Source: CAD feature listing. Evaluate the final solid. Frame: model axes, mm. A direction names the side the tool comes from. Give positions to 0.01 mm unless a question says otherwise; leave off trailing zeros. Order: outer loops, then holes, each group sorted by start corner. A loop starts at its lowest first (then second) coordinate and runs counter-clockwise, first axis right, second up. Notation, with made-up numbers: (10.5, 6.25) - (59.5, 6.25) arc R5 cw to (59.5, 14.25) - close; hole circle Ø7 at (78, 15.5). An arc over 180 degrees is marked (long way). One line per item, written item: value. Start each with the question number.
from build123d import *

# Parameters (mm, degrees)
SKETCH1_R           = 48.25
SKETCH1_R_2         = 36
BOSS_EXTRUDE6_DEPTH = 10
SKETCH21_R          = 2
CUT_EXTRUDE1_DEPTH  = 18
CIRPATTERN1_COUNT   = 8
SKETCH22_R          = 3.5
CUT_EXTRUDE2_DEPTH  = 4
CIRPATTERN2_COUNT   = 8
SKETCH23_R          = 48.25
BOSS_EXTRUDE7_DEPTH = 6
CUT_EXTRUDE3_START  = -6
SKETCH25_R          = 3.5
CUT_EXTRUDE3_DEPTH  = 6
CIRPATTERN4_COUNT   = 8


with BuildPart() as part:
    # Sketch1 → Boss-Extrude6 (new body)
    with BuildSketch(Plane(origin=(0, 0, 0), x_dir=(1, 0, 0), z_dir=(0, 1, 0))):
        with Locations(Location((0, 0, 0), (0, 0, 270))):
            Circle(SKETCH1_R)
        with Locations(Location((0, 0, 0), (0, 0, 270))):
            Circle(SKETCH1_R_2, mode=Mode.SUBTRACT)
    extrude(amount=BOSS_EXTRUDE6_DEPTH)

    # Sketch21 → Cut-Extrude1 (cut)
    with BuildSketch(Plane(origin=(0, 10, 0), x_dir=(1, 0, 0), z_dir=(0, 1, 0))):
        with Locations(Location((-42.5, 0, 0), (0, 0, 270))):
            Circle(SKETCH21_R)
    cut_extrude1 = extrude(amount=-CUT_EXTRUDE1_DEPTH, mode=Mode.SUBTRACT)

    # CirPattern1: Cut-Extrude1 ×8 about axis
    cirpattern1_axis = Axis((0, 0, 0), (0, 1, 0))
    for i in range(1, CIRPATTERN1_COUNT):
        add(cut_extrude1.rotate(cirpattern1_axis, i * 360 / CIRPATTERN1_COUNT), mode=Mode.SUBTRACT)

    # Sketch22 → Cut-Extrude2 (cut)
    with BuildSketch(Plane(origin=(0, 10, 0), x_dir=(1, 0, 0), z_dir=(0, 1, 0))):
        with Locations(Location((-42.5, 0, 0), (0, 0, 270))):
            Circle(SKETCH22_R)
    cut_extrude2 = extrude(amount=-CUT_EXTRUDE2_DEPTH, mode=Mode.SUBTRACT)

    # CirPattern2: Cut-Extrude2 ×8 about axis
    cirpattern2_axis = Axis((0, 0, 0), (0, 1, 0))
    for i in range(1, CIRPATTERN2_COUNT):
        add(cut_extrude2.rotate(cirpattern2_axis, i * 360 / CIRPATTERN2_COUNT), mode=Mode.SUBTRACT)

    # Sketch23 → Boss-Extrude7 (add)
    with BuildSketch(Plane(origin=(0, 10, 0), x_dir=(1, 0, 0), z_dir=(0, 1, 0))):
        with Locations(Location((0, 0, 0), (0, 0, 270))):
            Circle(SKETCH23_R)
    extrude(amount=BOSS_EXTRUDE7_DEPTH)

    # Sketch25 → Cut-Extrude3 (cut)
    with BuildSketch(Plane.XZ.offset(-10).offset(CUT_EXTRUDE3_START)):
        with Locations(Location((-42.5, 0, 0), (0, 0, 90))):
            Circle(SKETCH25_R)
    cut_extrude3 = extrude(amount=CUT_EXTRUDE3_DEPTH, mode=Mode.SUBTRACT)

    # CirPattern4: Cut-Extrude3 ×8 about axis
    cirpattern4_axis = Axis((0, 10, 0), (0, -1, 0))
    for i in range(1, CIRPATTERN4_COUNT):
        add(cut_extrude3.rotate(cirpattern4_axis, i * 360 / CIRPATTERN4_COUNT), mode=Mode.SUBTRACT)


solid = part.part
1. Section A-A on x = 0. Return the cut outline in (y, z), then the cut area to 3 significant figures.
2. Section B-B on z = 0. Return the cut outline in (x, y), then the cut area to 3 significant figures.
3. Set-up query: faces 4 (the flat face through (28, 6, -32)), 5 (the cylindrical face through (-0.923, 3.042, -44.274)), 6 (the cylindrical face through (10.81, 4.93, 34.34)). Return all of +Z, -Z, +X, -X, +Y, -Y with unobstructed straight access to the full face (end or side cutting, diameter ignored); none if empty.
4. Draft query along Z for faces 1 (the cylindrical face through (-47.103, 7.888, -10.46)), 2 (the flat face through (-36, 0, 7)), 3 (the flat face through (44, 6, -2)). Return one class per face: pulls with the +Z half, pulls with the -Z half, needs draft (parallel to the pull), parting line crosses it, or undercut.
5. Section D-D on y = 12.5. Count the separate pieces of the cut face and the enclosed holes in it, then the cut area to 3 significant figures.
6. Ray query, L1, parallel to X at y = 7, z = 31.5; L2, parallel to Z at x = 2.5, y = 2.5; L3, parallel to Z at x = -27, y = 4.5. Return the intervals inside material, ascending.
7. Section C-C on z = 42.5. Return the cut outline in (x, y), then the cut area to 3 significant figures.
8. Contact query for flat-ended pins moving along their axis: pin 1 Ø5.5 at (x, z) = (0.5, -42) entering from +Y; pin 2 Ø1.5 at (x, y) = (-29, 14.5) entering from +Z; pin 3 Ø4 at (y, z) = (14, -23) entering from -X. Output: stop coordinate, or through.
Data:
1. outline: (0, -48.25) - (16, -48.25) - (16, -46) - (6, -46) - (6, -44.5) - (0, -44.5) - close; (0, -40.5) - (6, -40.5) - (6, -39) - (16, -39) - (16, 39) - (6, 39) - (6, 40.5) - (0, 40.5) - (0, 36) - (10, 36) - (10, -36) - (0, -36) - close; (0, 44.5) - (6, 44.5) - (6, 46) - (16, 46) - (16, 48.25) - (0, 48.25) - close
1. area: 636 mm2
2. outline: (-48.25, 0) - (-44.5, 0) - (-44.5, 6) - (-46, 6) - (-46, 16) - (-48.25, 16) - close; (-40.5, 0) - (-36, 0) - (-36, 10) - (36, 10) - (36, 0) - (40.5, 0) - (40.5, 6) - (39, 6) - (39, 16) - (-39, 16) - (-39, 6) - (-40.5, 6) - close; (44.5, 0) - (48.25, 0) - (48.25, 16) - (46, 16) - (46, 6) - (44.5, 6) - close
2. area: 636 mm2
3. face 4: +Y
3. face 5: +Y, -Y
3. face 6: -Y
4. face 1: parting line crosses it
4. face 2: needs draft
4. face 3: undercut
5. separate pieces: 1
5. enclosed holes: 8
5. area: 7,010 mm2
6. L1: x = -36.55 to -33.24, -26.87 to -17.43, 17.43 to 26.87, 33.24 to 36.55
6. L2: z = -48.19 to -35.91, 35.91 to 48.19
6. L3: z = -39.99 to -23.81, 23.81 to 39.99
7. outline: (-22.84, 0) - (-2, 0) - (-2, 6) - (-3.5, 6) - (-3.5, 16) - (-22.84, 16) - close; (2, 0) - (22.84, 0) - (22.84, 16) - (3.5, 16) - (3.5, 6) - (2, 6) - close
7. area: 637 mm2
8. pin 1: stops at y = 6
8. pin 2: stops at z = 39.12
8. pin 3: stops at x = -43.44
